Geometry check sheet. Reference: drawing and pictorial views, mm from the part's lowest x, y, z. A direction names the side the tool comes from. Give positions to 0.01 mm unless a question says otherwise; leave off trailing zeros. Loops run counter-clockwise (first coordinate to the right, second up) from the corner with the lowest first, then second, coordinate; pieces in that order, holes last. Notation, with made-up numbers: (48.5, 14) -> (93.5, 14) arc R31 ccw to (93.5, 42) -> close; hole circle Ø10 at (37, 66). An arc over 180 degrees is marked (long way). Write item = value, one per line. Start each with the question number.
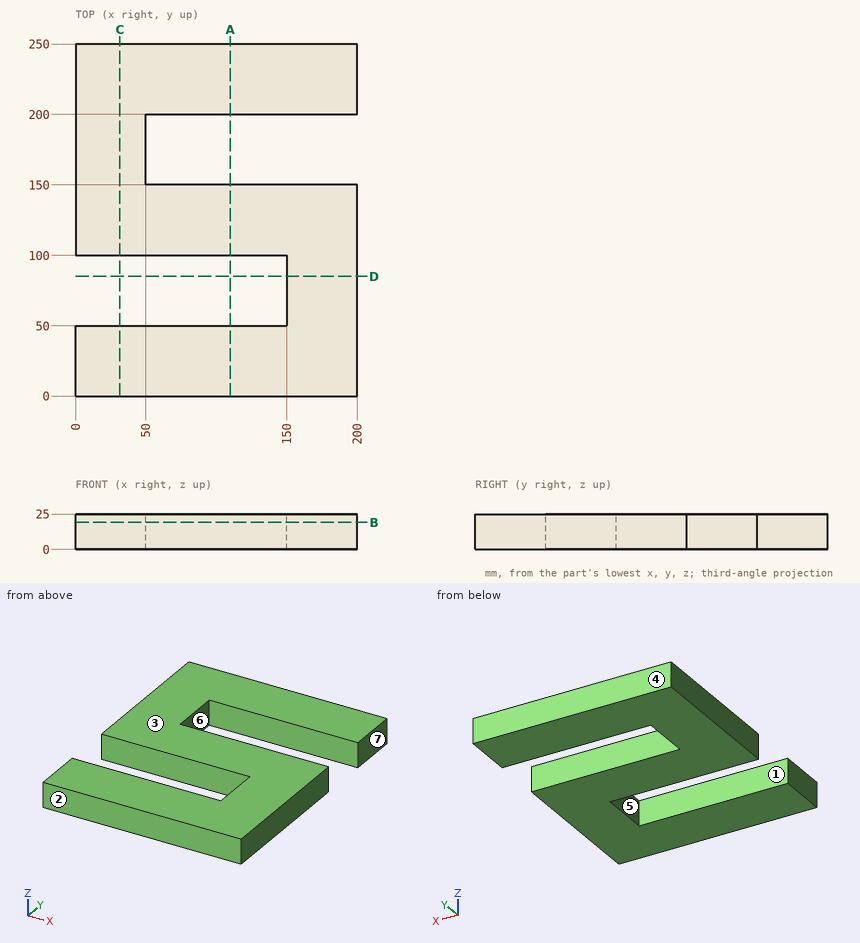
1) Draft check along Y on the marked faces 1, 2, 3 and 4. Enter one of: released by +Y, released by -Y, zero draft, split by the parting line, or undercut.
2) Depth check by flat-ended pin: pin 1 Ø4 at (y, z) = (187, 21.5) entering from +X; pin 2 Ø12.5 at (y, z) = (65, 13) entering from -X. Enter the tip coordinate at first touch or a pass-through.
3) Section check D-D (y = 85). Enter the section's corners in (x, z).
4) Section check B-B (z = 19.25). Enter the section's corners in (x, y).
5) Section check A-A (x = 110). Enter the section's corners in (y, z), plus the area to 3 significant figures.
6) Tool access check on the marked faces 5, 6 and 7. Record the directions out of +Z, -Z, +X, -X, +Y, -Y that give a thin tool (end or side, any length) a straight path to the whole face; none if there is none.
7) Section check C-C (x = 31.5). Enter the section's corners in (y, z).
8) Thickness scan on line 1 (Y direction, x = 65, z = 21.25); line 2 (Y direction, x = 169, z = 16.5); line 3 (Y direction, x = 38.5, z = 3.25). Record the ranges inside material, lowest first.
Check result:
q1.face_1 = undercut
q1.face_2 = released by -Y
q1.face_3 = zero draft
q1.face_4 = released by +Y
q2.pin_1 = 50
q2.pin_2 = 150
q3.outline = (150, 0) -> (200, 0) -> (200, 25) -> (150, 25) -> close
q4.outline = (0, 0) -> (200, 0) -> (200, 150) -> (50, 150) -> (50, 200) -> (200, 200) -> (200, 250) -> (0, 250) -> (0, 100) -> (150, 100) -> (150, 50) -> (0, 50) -> close
q5.outline = (0, 0) -> (50, 0) -> (50, 25) -> (0, 25) -> close; (100, 0) -> (150, 0) -> (150, 25) -> (100, 25) -> close; (200, 0) -> (250, 0) -> (250, 25) -> (200, 25) -> close
q5.area = 3,750 mm2
q6.face_5 = +Z, -Z, -X
q6.face_6 = +Z, -Z, +X
q6.face_7 = +Z, -Z, +X, +Y, -Y
q7.outline = (0, 0) -> (50, 0) -> (50, 25) -> (0, 25) -> close; (100, 0) -> (250, 0) -> (250, 25) -> (100, 25) -> close
q8.line_1 = 0 to 50, 100 to 150, 200 to 250
q8.line_2 = 0 to 150, 200 to 250
q8.line_3 = 0 to 50, 100 to 250
